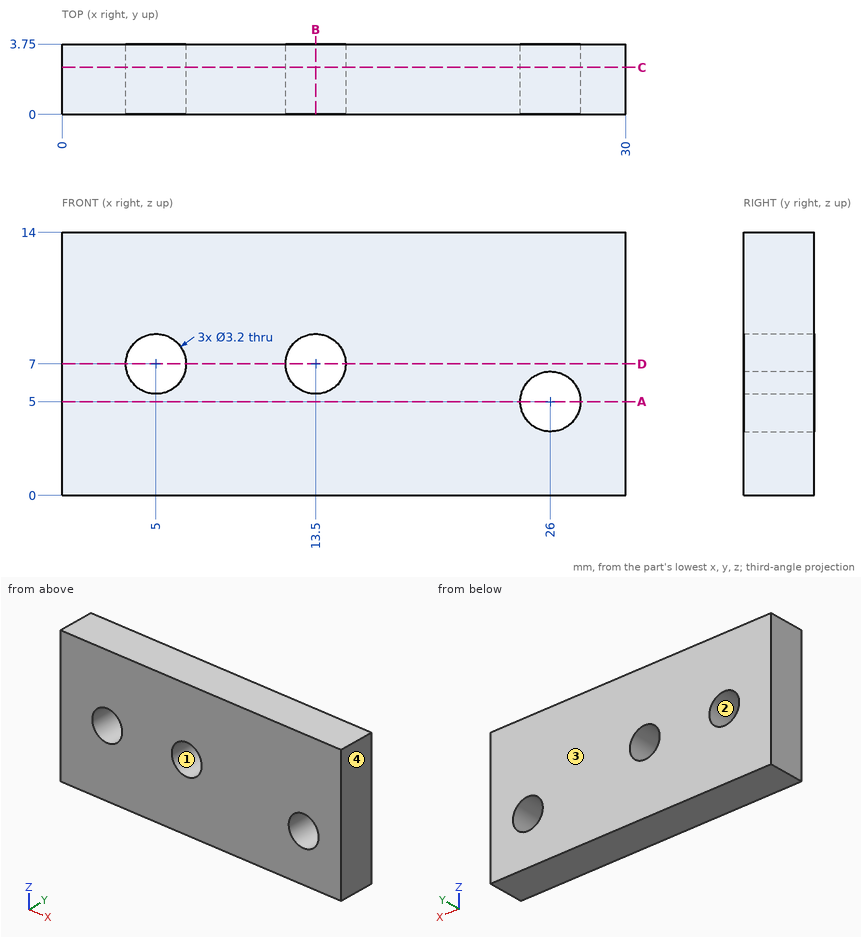
Geometry check sheet. Reference: drawing and pictorial views, mm from the part's lowest x, y, z. Give positions to 0.01 mm unless a question says otherwise; leave off trailing zeros. Loops run counter-clockwise (first coordinate to the right, second up) from the corner with the lowest first, then second, coordinate; pieces in that order, holes last. Notation, with made-up numbers: (70, -0.75) -> (79, -0.75) arc R7 cw to (79, 3.25) -> close; hole circle Ø9 at (-35.75, 26.25). An arc over 180 degrees is marked (long way). Answer in a Markdown table with one row per item. Add a question column.
1) Draft check along X on the marked faces 1, 2, 3 and 4. Enter one of: pulls with the +X half, pulls with the -X half, needs draft (parallel to the pull), parting line crosses it, or undercut.
2) Cross-section at A-A on z = 5. Record the boundary of the cut face in (x, y), and give its area (4 significant figures).
3) Cross-section at C-C on y = 2.5. Record the boundary of the cut face in (x, z), and give its area (3 significant figures).
4) Cross-section at D-D on z = 7. Record the boundary of the cut face in (x, y), and give its area (3 significant figures).
5) Material ranges on probe 1 along X at (y, z) = (2.9, 7); probe 2 along X at (y, z) = (2.75, 5); probe 3 along Z at (x, y) = (26, 3.05), recorded low to high. Write a range as from..to.
6) Cross-section at B-B on x = 13.5. Record the boundary of the cut face in (y, z), and give its area (3 significant figures).
Outcome:
| question | item | result |
|---|---|---|
| 1 | face 1 | undercut |
| 1 | face 2 | undercut |
| 1 | face 3 | needs draft |
| 1 | face 4 | pulls with the +X half |
| 2 | outline | (0, 0) -> (24.4, 0) -> (24.4, 3.75) -> (0, 3.75) -> close; (27.6, 0) -> (30, 0) -> (30, 3.75) -> (27.6, 3.75) -> close |
| 2 | area | 100.5 mm^2 |
| 3 | outline | (0, 0) -> (30, 0) -> (30, 14) -> (0, 14) -> close; hole circle Ø3.2 at (5, 7); hole circle Ø3.2 at (13.5, 7); hole circle Ø3.2 at (26, 5) |
| 3 | area | 396 mm^2 |
| 4 | outline | (0, 0) -> (3.4, 0) -> (3.4, 3.75) -> (0, 3.75) -> close; (6.6, 0) -> (11.9, 0) -> (11.9, 3.75) -> (6.6, 3.75) -> close; (15.1, 0) -> (30, 0) -> (30, 3.75) -> (15.1, 3.75) -> close |
| 4 | area | 88.5 mm^2 |
| 5 | probe 1 | x = 0..3.4, 6.6..11.9, 15.1..30 |
| 5 | probe 2 | x = 0..24.4, 27.6..30 |
| 5 | probe 3 | z = 0..3.4, 6.6..14 |
| 6 | outline | (0, 0) -> (3.75, 0) -> (3.75, 5.4) -> (0, 5.4) -> close; (0, 8.6) -> (3.75, 8.6) -> (3.75, 14) -> (0, 14) -> close |
| 6 | area | 40.5 mm^2 |
